Can you work these out from the model? Positions are in its coordinate system, mm. A direction names the side the tool comes from. Round coordinates to 2 decimals unless told otherwise and drop trailing zeros. Loops run counter-clockwise (first coordinate to the right, second up) from the corner with the lowest first, then second, coordinate; pieces in that order, holes last. Notation, with made-up numbers: (-3.75, 78.25) -> (38.25, 78.25) arc R14 ccw to (38.25, 88.25) -> close; hole circle Ø6 at (-2.5, -34.75). An arc over 180 degrees is marked (long way). Use a Markdown table: item, result.
from build123d import *

# Parameters (mm, degrees)
SKETCH_1_W           = 42
SKETCH_1_H           = 153
EXTRUDE_1_DEPTH      = 20
SKETCH_2_W           = 38
SKETCH_2_H           = 149
CUT_EXTRUDE_1_DEPTH  = 17
EXTRUDE_3_DEPTH      = 17
FILLET_START         = 2
FILLET_2_DEPTH       = 18
CHAMFER_1_SIZE       = 3
CUT_EXTRUDE_3_DEPTH  = 82.812285141
SKETCH_8_R           = 4
CUT_EXTRUDE_4_DEPTH  = 90.533513279
SKETCH_13_W          = 27
SKETCH_13_H          = 9.8440201
CUT_EXTRUDE_6_DEPTH  = 17
SKETCH_14_W          = 38
SKETCH_14_H          = 15.071373518
CUT_EXTRUDE_7_DEPTH  = 12.5
CUT_EXTRUDE_8_DEPTH  = 1
M3X0_51_D            = 2.5
M3X0_51_DEPTH        = 12.5
M3X0_51_TIP          = 0.751075774
M3X0_52_D            = 2.5
M3X0_52_DEPTH        = 12.5
M3X0_52_TIP          = 0.751075774
CUT_EXTRUDE_9_REACH  = 91.534
SKETCH_22_R          = 7.5
CUT_EXTRUDE_10_REACH = 91.534
SKETCH_23_R          = 4
CUT_EXTRUDE_11_REACH = 83.812
SKETCH_24_W          = 17
SKETCH_24_H          = 7
FILLET_3_R           = 1.5


with BuildPart() as part:
    # Эскиз1 → Бобышка-Вытянуть1 (new body)
    with BuildSketch(Plane.XY):
        Rectangle(SKETCH_1_W, SKETCH_1_H)
    extrude(amount=EXTRUDE_1_DEPTH)

    # Эскиз2 → Вырез-Вытянуть1 (cut)
    with BuildSketch(Plane.XY.offset(20)):
        Rectangle(SKETCH_2_W, SKETCH_2_H)
    extrude(amount=-CUT_EXTRUDE_1_DEPTH, mode=Mode.SUBTRACT)

    # Эскиз3 → Бобышка-Вытянуть3 (add)
    with BuildSketch(Plane.XY.offset(20)):
        with BuildLine():
            Line((-19, -71), (-19, -74.5))
            Line((-19, -74.5), (-15.5, -74.5))
            ThreePointArc((-15.5, -74.5), (-13.025126266, -68.525126266), (-19, -71))
        make_face()
        with BuildLine():
            Line((19, -71), (19, -74.5))
            Line((19, -74.5), (15.5, -74.5))
            ThreePointArc((15.5, -74.5), (13.025126266, -68.525126266), (19, -71))
        make_face()
        with BuildLine():
            Line((-15.5, 55), (-19, 55))
            Line((-19, 55), (-19, 48))
            Line((-19, 48), (-15.5, 48))
            ThreePointArc((-15.5, 48), (-12, 51.5), (-15.5, 55))
        make_face()
        with BuildLine():
            Line((15.5, 55), (19, 55))
            Line((19, 55), (19, 48))
            Line((19, 48), (15.5, 48))
            ThreePointArc((15.5, 48), (12, 51.5), (15.5, 55))
        make_face()
    extrude(amount=-EXTRUDE_3_DEPTH)

    # Скругление2: read off the stored shape, not the designer's step
    # Скругление2 outline → Скругление2 (add)
    with BuildSketch(Plane.XY.offset(FILLET_START)):
        with BuildLine():
            ThreePointArc((19, 58.983314774), (17.921186974, 56.25079457), (15.266666667, 54.992213561))
            ThreePointArc((15.266666667, 54.992213561), (15.383268392, 54.998052849), (15.5, 55))
            Line((15.5, 55), (19, 55))
            Line((19, 55), (19, 58.983314774))
        make_face()
        with BuildLine():
            ThreePointArc((15.5, 48), (15.383268392, 48.001947151), (15.266666667, 48.007786439))
            ThreePointArc((15.266666667, 48.007786439), (17.921186974, 46.74920543), (19, 44.016685226))
            Line((19, 44.016685226), (19, 48))
            Line((19, 48), (15.5, 48))
        make_face()
        with BuildLine():
            ThreePointArc((15, 74.5), (17.828427125, 73.328427125), (19, 70.5))
            Line((19, 70.5), (19, 74.5))
            Line((19, 74.5), (15, 74.5))
        make_face()
        with BuildLine():
            Line((19, -71), (19, -63.516685226))
            ThreePointArc((19, -63.516685226), (17.921186974, -66.24920543), (15.266666667, -67.507786439))
            ThreePointArc((15.266666667, -67.507786439), (17.890955179, -68.443961399), (19, -71))
        make_face()
        with BuildLine():
            ThreePointArc((-19, 70.5), (-17.828427125, 73.328427125), (-15, 74.5))
            Line((-15, 74.5), (-19, 74.5))
            Line((-19, 74.5), (-19, 70.5))
        make_face()
        with BuildLine():
            ThreePointArc((15.5, -74.5), (12.943961399, -73.390955179), (12.007786439, -70.766666667))
            ThreePointArc((12.007786439, -70.766666667), (10.74920543, -73.421186974), (8.016685226, -74.5))
            Line((8.016685226, -74.5), (15.5, -74.5))
        make_face()
        with BuildLine():
            ThreePointArc((-15.266666667, 54.992213561), (-17.921186974, 56.25079457), (-19, 58.983314774))
            Line((-19, 58.983314774), (-19, 55))
            Line((-19, 55), (-15.5, 55))
            ThreePointArc((-15.5, 55), (-15.383268392, 54.998052849), (-15.266666667, 54.992213561))
        make_face()
        with BuildLine():
            Line((-15.5, -74.5), (-8.016685226, -74.5))
            ThreePointArc((-8.016685226, -74.5), (-10.74920543, -73.421186974), (-12.007786439, -70.766666667))
            ThreePointArc((-12.007786439, -70.766666667), (-12.943961399, -73.390955179), (-15.5, -74.5))
        make_face()
        with BuildLine():
            ThreePointArc((-19, 44.016685226), (-17.921186974, 46.74920543), (-15.266666667, 48.007786439))
            ThreePointArc((-15.266666667, 48.007786439), (-15.383268392, 48.001947151), (-15.5, 48))
            Line((-15.5, 48), (-19, 48))
            Line((-19, 48), (-19, 44.016685226))
        make_face()
        with BuildLine():
            ThreePointArc((-19, -71), (-17.890955179, -68.443961399), (-15.266666667, -67.507786439))
            ThreePointArc((-15.266666667, -67.507786439), (-17.921186974, -66.24920543), (-19, -63.516685226))
            Line((-19, -63.516685226), (-19, -71))
        make_face()
    extrude(amount=FILLET_2_DEPTH)

    # Фаска1
    chamfer_1_edges = [part.edges().sort_by_distance(p)[0] for p in [
        (-21, 0, 0),
        (21, 0, 0),
    ]]
    chamfer(chamfer_1_edges, length=CHAMFER_1_SIZE)

    # Эскиз7 → Вырез-Вытянуть3 (cut, through all)
    with BuildSketch(Plane.XY.offset(20)):
        with BuildLine():
            Line((-21, -71), (-21, -76.5))
            Line((-21, -76.5), (-15.5, -76.5))
            ThreePointArc((-15.5, -76.5), (-19.389087297, -74.889087297), (-21, -71))
        make_face()
        with BuildLine():
            Line((21, -76.5), (15.5, -76.5))
            ThreePointArc((15.5, -76.5), (19.389087297, -74.889087297), (21, -71))
            Line((21, -71), (21, -76.5))
        make_face()
    extrude(amount=-CUT_EXTRUDE_3_DEPTH, mode=Mode.SUBTRACT)

    # Эскиз8 → Вырез-Вытянуть4 (cut, through all)
    with BuildSketch(Plane.ZY.offset(21)):
        with Locations((-3, -58.5)):
            Circle(SKETCH_8_R)
        with Locations((-3, -38.5)):
            Circle(SKETCH_8_R)
        with Locations((-3, -18.5)):
            Circle(SKETCH_8_R)
        with Locations((-3, 1.5)):
            Circle(SKETCH_8_R)
        with Locations((-3, 21.5)):
            Circle(SKETCH_8_R)
        with Locations((-3, 41.5)):
            Circle(SKETCH_8_R)
        with Locations((-3, 61.5)):
            Circle(SKETCH_8_R)
    extrude(amount=-CUT_EXTRUDE_4_DEPTH, mode=Mode.SUBTRACT)

    # Эскиз13 → Вырез-Вытянуть6 (cut)
    with BuildSketch(Plane.XY.offset(20)):
        with Locations((0, 76.5)):
            Rectangle(SKETCH_13_W, SKETCH_13_H)
    extrude(amount=-CUT_EXTRUDE_6_DEPTH, mode=Mode.SUBTRACT)

    # Эскиз14 → Вырез-Вытянуть7 (cut)
    with BuildSketch(Plane.XY.offset(20)):
        with Locations((0, 76.5)):
            Rectangle(SKETCH_14_W, SKETCH_14_H)
    extrude(amount=-CUT_EXTRUDE_7_DEPTH, mode=Mode.SUBTRACT)

    # Эскиз15 → Вырез-Вытянуть8 (cut)
    with BuildSketch(Plane.XY.offset(20)):
        with BuildLine():
            Line((-21, 76.5), (-21, -71))
            ThreePointArc((-21, -71), (-19.389087297, -74.889087297), (-15.5, -76.5))
            Line((-15.5, -76.5), (15.5, -76.5))
            ThreePointArc((15.5, -76.5), (19.389087297, -74.889087297), (21, -71))
            Line((21, -71), (21, 76.5))
            Line((21, 76.5), (20, 76.5))
            Line((20, 76.5), (20, -71))
            ThreePointArc((20, -71), (18.681980515, -74.181980515), (15.5, -75.5))
            Line((15.5, -75.5), (-15.5, -75.5))
            ThreePointArc((-15.5, -75.5), (-18.681980515, -74.181980515), (-20, -71))
            Line((-20, -71), (-20, 76.5))
            Line((-20, 76.5), (-21, 76.5))
        make_face()
    extrude(amount=-CUT_EXTRUDE_8_DEPTH, mode=Mode.SUBTRACT)

    # Отверстие обработанное метчиком M3x0.51
    with Locations(Plane.XY.offset(20)):
        with Locations((-15.5, 51.5), (15.5, 51.5), (15.5, -71), (-15.5, -71)):
            Hole(M3X0_51_D / 2, depth=M3X0_51_DEPTH)
            with Locations((0, 0, -(M3X0_51_DEPTH + M3X0_51_TIP / 2))):  # 118° drill point
                Cone(0, M3X0_51_D / 2, M3X0_51_TIP, mode=Mode.SUBTRACT)

    # Отверстие обработанное метчиком M3x0.52
    with Locations(Plane(origin=(0, 76.5, 0), x_dir=(1, 0, 0), z_dir=(0, 1, 0))):
        with Locations((-16.349186161, -4.77912666), (16.467977598, -4.67216637)):
            Hole(M3X0_52_D / 2, depth=M3X0_52_DEPTH)
            with Locations((0, 0, -(M3X0_52_DEPTH + M3X0_52_TIP / 2))):  # 118° drill point
                Cone(0, M3X0_52_D / 2, M3X0_52_TIP, mode=Mode.SUBTRACT)

    # Эскиз22 → Вырез-Вытянуть9 (cut, up to next)
    with BuildSketch(Plane(origin=(21, 0, 0), x_dir=(0, 0, -1), z_dir=(1, 0, 0)), mode=Mode.PRIVATE) as cut_extrude_9_sk1:
        with Locations((-19.5, 63.5)):
            Circle(SKETCH_22_R)
    cut_extrude_9_tool1 = extrude(cut_extrude_9_sk1.sketch, amount=-CUT_EXTRUDE_9_REACH, mode=Mode.PRIVATE) & part.part
    add(cut_extrude_9_tool1.solids().sort_by_distance((21, 63.5, 19.5))[0], mode=Mode.SUBTRACT)

    # Эскиз23 → Вырез-Вытянуть10 (cut, up to next)
    with BuildSketch(Plane.ZY.offset(21), mode=Mode.PRIVATE) as cut_extrude_10_sk1:
        with Locations((19.5, 67.89)):
            Circle(SKETCH_23_R)
    cut_extrude_10_tool1 = extrude(cut_extrude_10_sk1.sketch, amount=-CUT_EXTRUDE_10_REACH, mode=Mode.PRIVATE) & part.part
    add(cut_extrude_10_tool1.solids().sort_by_distance((-21, 67.89, 19.5))[0], mode=Mode.SUBTRACT)

    # Эскиз24 → Вырез-Вытянуть11 (cut, up to next)
    with BuildSketch(Plane(origin=(0, 0, 0), x_dir=(-1, 0, 0), z_dir=(0, 0, -1)), mode=Mode.PRIVATE) as cut_extrude_11_sk1:
        with Locations((0, 69)):
            Rectangle(SKETCH_24_W, SKETCH_24_H)
    cut_extrude_11_tool1 = extrude(cut_extrude_11_sk1.sketch, amount=-CUT_EXTRUDE_11_REACH, mode=Mode.PRIVATE) & part.part
    add(cut_extrude_11_tool1.solids().sort_by_distance((0, 69, 0))[0], mode=Mode.SUBTRACT)

    # Скругление3
    fillet_3_edges = [part.edges().sort_by_distance(p)[0] for p in [
        (-8.5, 72.5, 1.5),
        (-8.5, 65.5, 1.5),
        (8.5, 65.5, 1.5),
        (8.5, 72.5, 1.5),
    ]]
    fillet(fillet_3_edges, radius=FILLET_3_R)


solid = part.part
1. Will these pins go through, and if not, where does the flat tip stop? pin 1 Ø2 at (x, y) = (15.5, 51.5) entering from +Z; pin 2 Ø1.5 at (x, y) = (6, 9) entering from +Z; pin 3 Ø6 at (x, y) = (-15.5, 75) entering from +Z.
Answer sheet:
| item | result |
|---|---|
| pin 1 | stops at z = 7.35 |
| pin 2 | stops at z = 3 |
| pin 3 | stops at z = 7.5 |
2. Which directions (+Z, -Z, +X, -X, +Y, -Y) give clear straight access to the entire face, cutting with the end or side of a thin tool? Please do faces 1 (the cylindrical face through (17.95, 56.28, 9.49)), 2 (the cylindrical face through (18.717, -74.147, 19.507)), 3 (the flat face through (0, -74.5, 12)).
Answer sheet:
| item | result |
|---|---|
| face 1 | +Z |
| face 2 | +Z, +X, -Y |
| face 3 | +Z, +Y |
3. I need wall thicknesses on line 1 (X direction, y = 51.5, z = 15.25); line 2 (Y direction, x = 15.5, z = 13); line 3 (Y direction, x = -4.5, z = 1.25). Which ranges of each line are inside material? Lowest first, please.
Answer sheet:
| item | result |
|---|---|
| line 1 | x = -21 to -16.75, -14.25 to -12, 12 to 14.25, 16.75 to 21 |
| line 2 | y = -76.5 to -72.25, -69.75 to -67.49, 47.99 to 50.25, 52.75 to 55.01 |
| line 3 | y = -76.5 to 65.5, 72.5 to 76.5 |
4. If we mould it in two halves opening along X, with no side actions, what happens to faces 4 (the flat face through (-21, 2, 11)), 5 (the flat face through (19, 68, 10)), 6 (the cylindrical face through (18.25, 72.83, 5.22)), 7 (the cylindrical face through (-0.3, -18.5, 1))? For each: +X half, -X half, draft (parallel to the pull), parting line (faces both ways), or undercut.
Answer sheet:
| item | result |
|---|---|
| face 4 | -X half |
| face 5 | undercut |
| face 6 | undercut |
| face 7 | draft |
5. I want a section at A-A (x = -0.5). Please give me the cut outline in (y, z).
Answer sheet:
| item | result |
|---|---|
| outline | (-76.5, 0) -> (-61.15, 0) arc R4 cw to (-55.85, 0) -> (-41.15, 0) arc R4 cw to (-35.85, 0) -> (-21.15, 0) arc R4 cw to (-15.85, 0) -> (-1.15, 0) arc R4 cw to (4.15, 0) -> (18.85, 0) arc R4 cw to (24.15, 0) -> (38.85, 0) arc R4 cw to (44.15, 0) -> (58.85, 0) arc R4 cw to (64.15, 0) -> (65.5, 0) -> (65.5, 3) -> (-74.5, 3) -> (-74.5, 20) -> (-75.5, 20) -> (-75.5, 19) -> (-76.5, 19) -> close; (72.5, 0) -> (76.5, 0) -> (76.5, 3) -> (72.5, 3) -> close |
